```python
from build123d import *

# Parameters (mm, degrees)
SKETCH1_W           = 40
SKETCH1_H           = 36
BOSS_EXTRUDE1_DEPTH = 8
SKETCH2_R           = 6
CUT_EXTRUDE1_DEPTH  = 55.405882035
SKETCH3_W           = 20
SKETCH3_H           = 3.4
CUT_EXTRUDE2_DEPTH  = 55.405882035
SKETCH6_R           = 1.45
CUT_EXTRUDE3_DEPTH  = 55.405882035
SKETCH7_R           = 6.5
SKETCH7_W           = 14
SKETCH7_H           = 13
CUT_EXTRUDE4_DEPTH  = 55.405882035


with BuildPart() as part:
    # Sketch1 → Boss-Extrude1 (new body)
    with BuildSketch(Plane(origin=(0, 0, 0), x_dir=(0, 0, -1), z_dir=(1, 0, 0))):
        with Locations((20, -18)):
            Rectangle(SKETCH1_W, SKETCH1_H)
    extrude(amount=BOSS_EXTRUDE1_DEPTH)

    # Sketch2 → Cut-Extrude1 (cut, through all)
    with BuildSketch(Plane(origin=(8, 0, 0), x_dir=(0, 0, -1), z_dir=(1, 0, 0))):
        with Locations((20, -18)):
            Circle(SKETCH2_R)
    extrude(amount=-CUT_EXTRUDE1_DEPTH, mode=Mode.SUBTRACT)

    # Sketch3 → Cut-Extrude2 (cut, through all)
    with BuildSketch(Plane(origin=(8, 0, 0), x_dir=(0, 0, -1), z_dir=(1, 0, 0))):
        with Locations((20, -5.5)):
            Rectangle(SKETCH3_W, SKETCH3_H)
        with Locations((20, -30.5)):
            Rectangle(SKETCH3_W, SKETCH3_H)
    extrude(amount=-CUT_EXTRUDE2_DEPTH, mode=Mode.SUBTRACT)

    # Sketch6 → Cut-Extrude3 (cut, through all)
    with BuildSketch(Plane(origin=(0, 0, 0), x_dir=(1, 0, 0), z_dir=(0, 1, 0))):
        with Locations(Location((4, 4, 0), (0, 0, 270))):
            Circle(SKETCH6_R)
        with Locations(Location((4, 36, 0), (0, 0, 270))):
            Circle(SKETCH6_R)
    extrude(amount=-CUT_EXTRUDE3_DEPTH, mode=Mode.SUBTRACT)

    # Sketch7 → Cut-Extrude4 (cut, through all)
    with BuildSketch(Plane(origin=(8, 0, 0), x_dir=(0, 0, -1), z_dir=(1, 0, 0))):
        with Locations((27, -18)):
            Circle(SKETCH7_R)
        with Locations((13, -18)):
            Circle(SKETCH7_R)
        with Locations((20, -18)):
            Rectangle(SKETCH7_W, SKETCH7_H)
    extrude(amount=-CUT_EXTRUDE4_DEPTH, mode=Mode.SUBTRACT)


solid = part.part
```
Could you check a few things on this model? Use its own coordinates, in mm. A direction names the side the tool comes from. Coordinates: 2 decimals unless noted, no trailing zeros. Loops run counter-clockwise (first coordinate to the right, second up) from the corner with the lowest first, then second, coordinate; pieces in that order, holes last.
1) Please list where these lines run through material, in increasing order: line 1 along Y through (x, z) = (5.75, -21); line 2 along X through (y, z) = (-28, -4); line 3 along Z through (x, y) = (7.5, -6).
Reported:
line 1: y = -36 to -32.2, -28.8 to -24.5, -11.5 to -7.2, -3.8 to 0
line 2: x = 0 to 2.55, 5.45 to 8
line 3: z = -40 to -30, -10 to 0
2) Which directions (+Z, -Z, +X, -X, +Y, -Y) give clear straight access to the entire face, cutting with the end or side of a thin tool? Please do faces 1 (the face through (4, -24.5, -20)), 2 (the face through (4, -18, 0)).
Reported:
face 1: +X, -X
face 2: +Z, +X, -X, +Y, -Y
3) Imagine slicing it at D-D (x = 6.75). List the corners of the cut face in (y, z) for me.
Reported:
outline: (-36, -40) - (0, -40) - (0, 0) - (-36, 0) - close; hole (-32.2, -30) - (-28.8, -30) - (-28.8, -10) - (-32.2, -10) - close; hole (-24.5, -27) arc R6.5 ccw to (-11.5, -27) - (-11.5, -13) arc R6.5 ccw to (-24.5, -13) - close; hole (-7.2, -30) - (-3.8, -30) - (-3.8, -10) - (-7.2, -10) - close
4) Thinking about a two-plate mould opening in Y: for faces 3 (the face through (4, 0, -20)), 4 (the face through (4, -11.5, -20)), 5 (the face through (3.12, -17.75, -5.15)), which applies, released by +Y, released by -Y, zero draft, split by the parting line, or undercut?
Reported:
face 3: released by +Y
face 4: undercut
face 5: zero draft
5) Imagine slicing it at A-A (x = 4). List the corners of the cut face in (y, z) for me, and give its area (3 significant figures).
Reported:
outline: (-36, -40) - (0, -40) - (0, -37.45) - (-36, -37.45) - close; (-36, -34.55) - (0, -34.55) - (0, -5.45) - (-36, -5.45) - close; (-36, -2.55) - (0, -2.55) - (0, 0) - (-36, 0) - close; hole (-32.2, -30) - (-28.8, -30) - (-28.8, -10) - (-32.2, -10) - close; hole (-24.5, -27) arc R6.5 ccw to (-11.5, -27) - (-11.5, -13) arc R6.5 ccw to (-24.5, -13) - close; hole (-7.2, -30) - (-3.8, -30) - (-3.8, -10) - (-7.2, -10) - close
area: 780 mm2
6) Imagine slicing it at C-C (z = -36). List the corners of the cut face in (x, y) for me.
Reported:
outline: (0, -36) - (2.55, -36) - (2.55, 0) - (0, 0) - close; (5.45, -36) - (8, -36) - (8, 0) - (5.45, 0) - close
7) Imagine slicing it at B-B (y = -18). List the corners of the cut face in (x, z) for me, and give its area (3 significant figures).
Reported:
outline: (0, -40) - (8, -40) - (8, -33.5) - (0, -33.5) - close; (0, -6.5) - (8, -6.5) - (8, 0) - (0, 0) - close; hole circle Ø2.9 at (4, -36); hole circle Ø2.9 at (4, -4)
area: 90.8 mm2
